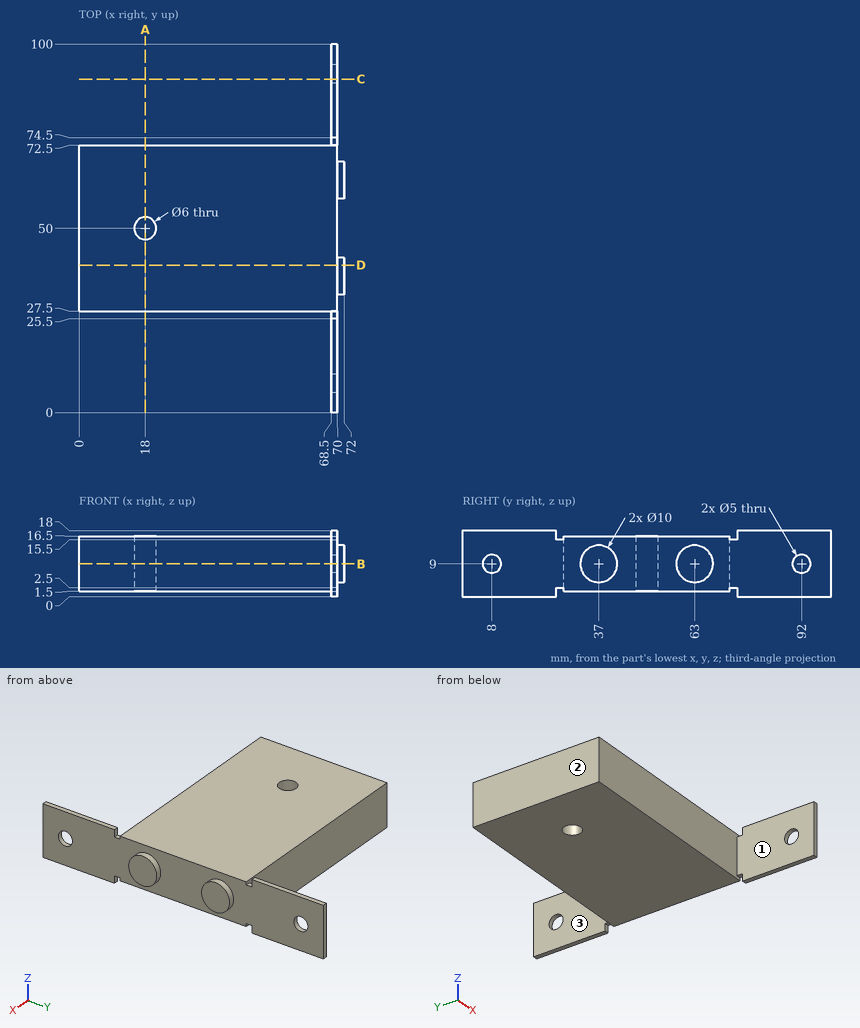
Study the drawing (mm; zero at the part's minimum x, y, z) and answer. A direction names the side the tool comes from. Give positions to 0.01 mm unless a question says otherwise; leave off trailing zeros. Loops run counter-clockwise (first coordinate to the right, second up) from the corner with the lowest first, then second, coordinate; pieces in that order, holes last. Notation, with made-up numbers: (-8, 18.5) - (11, 18.5) arc R15 ccw to (11, 34.5) - close; hole circle Ø7 at (42, 88). An arc over 180 degrees is marked (long way). Return JSON: item names as keys, results as strings. Group by question number.
1. Given pin 1 Ø5.5 at (y, z) = (19, 10.5) entering from -X; pin 2 Ø5 at (y, z) = (45, 15) entering from +X; pin 3 Ø0.8 at (x, y) = (69, 26) entering from +Z, each flat-ended and moving along its own axis, determine where each tip first touches the part or whether it passes through.
2. Find section C-C (y = 90.5). Write down the section's boundary in (x, z), then the cut area to 3 significant figures.
3. Find section B-B (z = 9). Write down the section's boundary in (x, y), then the cut area to 3 significant figures.
4. Find section A-A (x = 18). Write down the section's boundary in (y, z), then the cut area to 3 significant figures.
5. Straight lines are drawn through the part: line 1 (Y direction, x = 69.2, z = 9); line 2 (Y direction, x = 18, z = 13.5); line 3 (Y direction, x = 12, z = 16.25). For each, find the intervals that lie inside material, in ascending order. Write a range as [from, to].
6. Which of the six approach directions +Z, -Z, +X, -X, +Y, -Y give full straight-line access (tool end or side, diameter ignored) to the marked faces 1, 2 and 3?
7. Find section D-D (y = 40). Write down the section's boundary in (x, z).
Verdict:
{
 "1": {"pin 1": "stops at x = 68.5", "pin 2": "stops at x = 70", "pin 3": "stops at z = 15.5"},
 "2": {"outline": "(68.5, 0) - (70, 0) - (70, 7) - (68.5, 7) - close; (68.5, 11) - (70, 11) - (70, 18) - (68.5, 18) - close", "area": "21.0 mm^2"},
 "3": {"outline": "(0, 27.5) - (68.5, 27.5) - (68.5, 10.5) - (70, 10.5) - (70, 32) - (72, 32) - (72, 42) - (70, 42) - (70, 58) - (72, 58) - (72, 68) - (70, 68) - (70, 89.5) - (68.5, 89.5) - (68.5, 72.5) - (0, 72.5) - close; (68.5, 0) - (70, 0) - (70, 5.5) - (68.5, 5.5) - close; (68.5, 94.5) - (70, 94.5) - (70, 100) - (68.5, 100) - close; hole circle Ø6 at (18, 50)", "area": "3,230 mm^2"},
 "4": {"outline": "(27.5, 1.5) - (47, 1.5) - (47, 16.5) - (27.5, 16.5) - close; (53, 1.5) - (72.5, 1.5) - (72.5, 16.5) - (53, 16.5) - close", "area": "585 mm^2"},
 "5": {"line 1": "y = [0, 5.5], [10.5, 89.5], [94.5, 100]", "line 2": "y = [27.5, 47], [53, 72.5]", "line 3": "y = [27.5, 72.5]"},
 "6": {"face 1": "+Z, -Z, -X, -Y", "face 2": "+Z, -Z, -X, +Y, -Y", "face 3": "+Z, -Z, -X, +Y"},
 "7": {"outline": "(0, 1.5) - (70, 1.5) - (70, 5) - (72, 5) - (72, 13) - (70, 13) - (70, 16.5) - (0, 16.5) - close"}
}
